Geometry: final body of the model. Coordinates: model frame, mm. Face numbers are marked on the shaded views. A direction names the side the tool comes from. Round coordinates to 2 decimals unless told otherwise and drop trailing zeros. Loops run counter-clockwise (first coordinate to the right, second up) from the corner with the lowest first, then second, coordinate; pieces in that order, holes last. Notation, with made-up numbers: (-38, -30) -> (-27, -30) arc R27 ccw to (-27, 1) -> close; hole circle Ø2 at (88.5, 18.5). An arc over 180 degrees is marked (long way). Answer in a Markdown table with one row per item.
```python
from build123d import *

# Parameters (mm, degrees)
SKETCH2_R           = 25
BOSS_EXTRUDE2_DEPTH = 30
CUT_EXTRUDE2_START  = -30
CUT_EXTRUDE2_DEPTH  = 30
SKETCH4_R           = 3.19
CUT_EXTRUDE3_DEPTH  = 30


with BuildPart() as part:
    # Sketch2 → Boss-Extrude2 (new body)
    with BuildSketch(Plane.XY):
        Circle(SKETCH2_R)
    extrude(amount=BOSS_EXTRUDE2_DEPTH)

    # Sketch3 → Cut-Extrude2 (cut)
    with BuildSketch(Plane.XY.offset(30).offset(CUT_EXTRUDE2_START)):
        with BuildLine():
            Line((6.913843876, -7.224871131), (17.934101996, -13.587420123))
            ThreePointArc((17.934101996, -13.587420123), (15.608801126, -16.205410436), (12.905469818, -18.430920997))
            Line((12.905469818, -18.430920997), (14.339410909, -20.478801107))
            ThreePointArc((14.339410909, -20.478801107), (12.5, -21.650635095), (10.565456544, -22.657694676))
            Line((10.565456544, -22.657694676), (9.508910889, -20.391925208))
            ThreePointArc((9.508910889, -20.391925208), (6.229896553, -21.620323516), (2.8, -22.325097984))
            Line((2.8, -22.325097984), (2.8, -9.6))
            ThreePointArc((2.8, -9.6), (5, -8.660254038), (6.913843876, -7.224871131))
        make_face()
        with BuildLine():
            Line((9.713843876, -2.375128869), (20.734101996, -8.737677861))
            ThreePointArc((20.734101996, -8.737677861), (21.83869768, -5.41491308), (22.414380707, -1.961004212))
            Line((22.414380707, -1.961004212), (24.904867452, -2.178893569))
            ThreePointArc((24.904867452, -2.178893569), (25, 0), (24.904867452, 2.178893569))
            Line((24.904867452, 2.178893569), (22.414380707, 1.961004212))
            ThreePointArc((22.414380707, 1.961004212), (21.83869768, 5.41491308), (20.734101996, 8.737677861))
            Line((20.734101996, 8.737677861), (9.713843876, 2.375128869))
            ThreePointArc((9.713843876, 2.375128869), (10, 0), (9.713843876, -2.375128869))
        make_face()
        with BuildLine():
            Line((-2.8, -9.6), (-2.8, -22.325097984))
            ThreePointArc((-2.8, -22.325097984), (-6.229896553, -21.620323516), (-9.508910889, -20.391925208))
            Line((-9.508910889, -20.391925208), (-10.565456544, -22.657694676))
            ThreePointArc((-10.565456544, -22.657694676), (-12.5, -21.650635095), (-14.339410909, -20.478801107))
            Line((-14.339410909, -20.478801107), (-12.905469818, -18.430920997))
            ThreePointArc((-12.905469818, -18.430920997), (-15.608801126, -16.205410436), (-17.934101996, -13.587420123))
            Line((-17.934101996, -13.587420123), (-6.913843876, -7.224871131))
            ThreePointArc((-6.913843876, -7.224871131), (-5, -8.660254038), (-2.8, -9.6))
        make_face()
        with BuildLine():
            Line((-9.713843876, -2.375128869), (-20.734101996, -8.737677861))
            ThreePointArc((-20.734101996, -8.737677861), (-21.83869768, -5.41491308), (-22.414380707, -1.961004212))
            Line((-22.414380707, -1.961004212), (-24.904867452, -2.178893569))
            ThreePointArc((-24.904867452, -2.178893569), (-25, 0), (-24.904867452, 2.178893569))
            Line((-24.904867452, 2.178893569), (-22.414380707, 1.961004212))
            ThreePointArc((-22.414380707, 1.961004212), (-21.83869768, 5.41491308), (-20.734101996, 8.737677861))
            Line((-20.734101996, 8.737677861), (-9.713843876, 2.375128869))
            ThreePointArc((-9.713843876, 2.375128869), (-10, 0), (-9.713843876, -2.375128869))
        make_face()
        with BuildLine():
            Line((-6.913843876, 7.224871131), (-17.934101996, 13.587420123))
            ThreePointArc((-17.934101996, 13.587420123), (-15.608801126, 16.205410436), (-12.905469818, 18.430920997))
            Line((-12.905469818, 18.430920997), (-14.339410909, 20.478801107))
            ThreePointArc((-14.339410909, 20.478801107), (-12.5, 21.650635095), (-10.565456544, 22.657694676))
            Line((-10.565456544, 22.657694676), (-9.508910889, 20.391925208))
            ThreePointArc((-9.508910889, 20.391925208), (-6.229896553, 21.620323516), (-2.8, 22.325097984))
            Line((-2.8, 22.325097984), (-2.8, 9.6))
            ThreePointArc((-2.8, 9.6), (-5, 8.660254038), (-6.913843876, 7.224871131))
        make_face()
        with BuildLine():
            Line((2.8, 9.6), (2.8, 22.325097984))
            ThreePointArc((2.8, 22.325097984), (6.229896553, 21.620323516), (9.508910889, 20.391925208))
            Line((9.508910889, 20.391925208), (10.565456544, 22.657694676))
            ThreePointArc((10.565456544, 22.657694676), (12.5, 21.650635095), (14.339410909, 20.478801107))
            Line((14.339410909, 20.478801107), (12.905469818, 18.430920997))
            ThreePointArc((12.905469818, 18.430920997), (15.608801126, 16.205410436), (17.934101996, 13.587420123))
            Line((17.934101996, 13.587420123), (6.913843876, 7.224871131))
            ThreePointArc((6.913843876, 7.224871131), (5, 8.660254038), (2.8, 9.6))
        make_face()
    extrude(amount=CUT_EXTRUDE2_DEPTH, mode=Mode.SUBTRACT)

    # Sketch4 → Cut-Extrude3 (cut)
    with BuildSketch(Plane.XY.offset(30)):
        Circle(SKETCH4_R)
    extrude(amount=-CUT_EXTRUDE3_DEPTH, mode=Mode.SUBTRACT)


solid = part.part
```
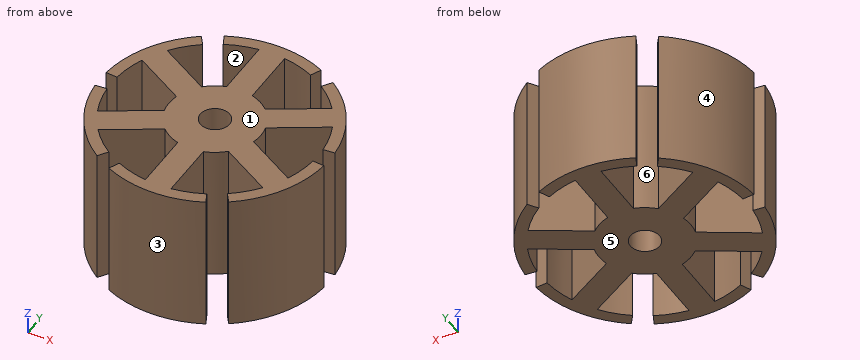
Item 1: Section query B-B, the plane x = 0. Output: boundary loops of the cut face in (y, z).
Ans:
| item | result |
|---|---|
| outline | (-25, 0) -> (-3.19, 0) -> (-3.19, 30) -> (-25, 30) -> close; (3.19, 0) -> (25, 0) -> (25, 30) -> (3.19, 30) -> close |
Item 2: Section query A-A, the plane y = 0. Output: boundary loops of the cut face in (x, z).
Ans:
| item | result |
|---|---|
| outline | (-10, 0) -> (-3.19, 0) -> (-3.19, 30) -> (-10, 30) -> close; (3.19, 0) -> (10, 0) -> (10, 30) -> (3.19, 30) -> close |
Item 3: Ray query, L1, parallel to Y at x = -7, z = 20.75; L2, parallel to Y at x = 4, z = 7; L3, parallel to X at y = 17, z = 21. Return the intervals inside material, ascending.
Ans:
| item | result |
|---|---|
| L1 | -24 to -21.38, -7.27 to 7.27, 21.38 to 24 |
| L2 | -24.68 to -22.14, -9.17 to 9.17, 22.14 to 24.68 |
| L3 | -18.33 to -14.74, -2.8 to 2.8, 14.74 to 18.33 |
Item 4: Set-up query: the marked faces 5 and 6. Return all of +Z, -Z, +X, -X, +Y, -Y with unobstructed straight access to the full face (end or side cutting, diameter ignored); none if empty.
Ans:
| item | result |
|---|---|
| face 5 | -Z, +X, -X, +Y, -Y |
| face 6 | +Z, -Z |
Item 5: Section query C-C, the plane y = 19.5. Output: boundary loops of the cut face in (x, z).
Ans:
| item | result |
|---|---|
| outline | (-15.64, 0) -> (-13.65, 0) -> (-13.65, 30) -> (-15.64, 30) -> close; (-2.8, 0) -> (2.8, 0) -> (2.8, 30) -> (-2.8, 30) -> close; (13.65, 0) -> (15.64, 0) -> (15.64, 30) -> (13.65, 30) -> close |
Item 6: First-contact query: P1, Ø14, axis at y = -17, z = 12.5, coming from the +X side; P2, Ø12, axis at x = -17.5, y = -18.5, coming from the +Z side; P3, Ø4, axis at y = 15, z = 14, coming from the +X side; P4, Ø4, axis at y = 7, z = 12, coming from the -X side. Flat tips, straight axial feed; report the tip coordinate or a pass-through.
Ans:
| item | result |
|---|---|
| P1 | x = 22.91 |
| P2 | z = 30 |
| P3 | x = 21.35 |
| P4 | x = -24.49 |
Item 7: Mould query, pull axis X, two halves, no side actions, for the marked faces 1, 2, 3 and 4. Classes: released by +X, released by -X, zero draft, split by the parting line, or undercut.
Ans:
| item | result |
|---|---|
| face 1 | zero draft |
| face 2 | undercut |
| face 3 | split by the parting line |
| face 4 | released by -X |
